```python
from build123d import *

# Parameters (mm, degrees)
CYLINDER093_R     = 5
CYLINDER093_DEPTH = 8.8
CYLINDER092_R     = 10
CYLINDER092_DEPTH = 2.8
CHAMFER004_SIZE   = 0.75


with BuildPart() as cylinder093:
    # Cylinder093 → Cylinder093 (new body)
    with BuildSketch(Plane.XY.offset(12)):
        Circle(CYLINDER093_R)
    extrude(amount=CYLINDER093_DEPTH)


with BuildPart() as hub_rear_support:
    # Cylinder092 → Cylinder092 (new body)
    with BuildSketch(Plane.XY.offset(12)):
        Circle(CYLINDER092_R)
    extrude(amount=CYLINDER092_DEPTH)

    # Fusion047: union Cylinder093
    add(cylinder093.part)

    # Chamfer004
    chamfer004_edges = [hub_rear_support.edges().sort_by_distance(p)[0] for p in [
        (-10, 0, 12),
    ]]
    chamfer(chamfer004_edges, length=CHAMFER004_SIZE)


solid = hub_rear_support.part
```
Work out the finished part from the listing and answer in its coordinate system (mm). A direction names the side the tool comes from. Round coordinates to 2 decimals unless told otherwise and drop trailing zeros. Order: outer loops, then holes, each group sorted by start corner. A loop starts at its lowest first (then second) coordinate and runs counter-clockwise, first axis right, second up.
Q1. A cutting plane is placed at C-C, the plane z = 13.5. Determine the outline of the cut face in (x, y).
Solution:
outline: circle Ø20 at (0, 0)
Q2. A cutting plane is placed at D-D, the plane z = 18. Determine the outline of the cut face in (x, y), then the cut area to 3 significant figures.
Solution:
outline: circle Ø10 at (0, 0)
area: 78.5 mm2
Q3. A tool of negligible diameter and unlimited length cuts with its end or side. For faces 1 (the cylindrical face through (-1.08, -4.88, 17.76)), 2 (the flat face through (0, 0, 12)), from which of +Z, -Z, +X, -X, +Y, -Y can it reach the whole face along a straight path? Write none if from no direction.
Solution:
face 1: +Z
face 2: -Z, +X, -X, +Y, -Y
Q4. Find the intervals of material crossed by line 1 along Z through (x, y) = (1.25, 8.75); line 2 along Y through (x, z) = (0.5, 15); line 3 along X through (y, z) = (2.25, 18), in increasing order.
Solution:
line 1: z = 12 to 14.8
line 2: y = -4.97 to 4.97
line 3: x = -4.47 to 4.47
Q5. Given pin 1 Ø3 at (x, z) = (-2.5, 19) entering from +Y; pin 2 Ø3 at (x, y) = (7.5, 4) entering from +Z, each flat-ended and moving along its own axis, determine where each tip first touches the part or whether it passes through.
Solution:
pin 1: stops at y = 4.9
pin 2: stops at z = 14.8
Q6. A cutting plane is placed at A-A, the plane x = 0. Determine the outline of the cut face in (y, z), then the cut area to 3 significant figures.
Solution:
outline: (-10, 12.75) - (-9.25, 12) - (9.25, 12) - (10, 12.75) - (10, 14.8) - (5, 14.8) - (5, 20.8) - (-5, 20.8) - (-5, 14.8) - (-10, 14.8) - close
area: 115 mm2
